Design review of the part built by this model. Coordinates are the model's own, in mm. Face numbers are marked on the shaded views. A direction names the side the tool comes from. Round coordinates to 2 decimals unless told otherwise and drop trailing zeros. Loops run counter-clockwise (first coordinate to the right, second up) from the corner with the lowest first, then second, coordinate; pieces in that order, holes last. Notation, with made-up numbers: (37, 69) - (90, 69) arc R31 ccw to (90, 97) - close; hole circle Ø4 at (-38, 5.5). An arc over 180 degrees is marked (long way). Answer as CSV lines item,"result". Start each with the question number.
(1) Wall thickness on L1, parallel to Z at x = 24.75, y = 7.25; L2, parallel to X at y = 1.5, z = -2; L3, parallel to X at y = 1.5, z = -66.5: over which ranges is each line inside the solid? List them lowest first.
(2) For P1, Ø2, axis at x = 9.5, y = 3, coming from the -Z side; P2, Ø3, axis at y = 4, z = -44.5, coming from the +X side; P3, Ø2, axis at y = 5, z = -30.5, coming from the -X side, all flat-tipped, find the tip position at first contact; note any pin that passes through.
(3) Consider section B-B (z = 2). Give the boundary of the cut face in (x, y).
(4) Consider section C-C (x = 24). Give the boundary of the cut face in (y, z).
(5) For the marked faces 1 and 2, list the 3-axis set-ups (+Z, -Z, +X, -X, +Y, -Y) from which the entire face can be reached by the end or side of a thin tool; tool diameter is ignored.
(6) Consider section A-A (y = 4.5). Give the boundary of the cut face in (x, z), and give its area (3 significant figures).
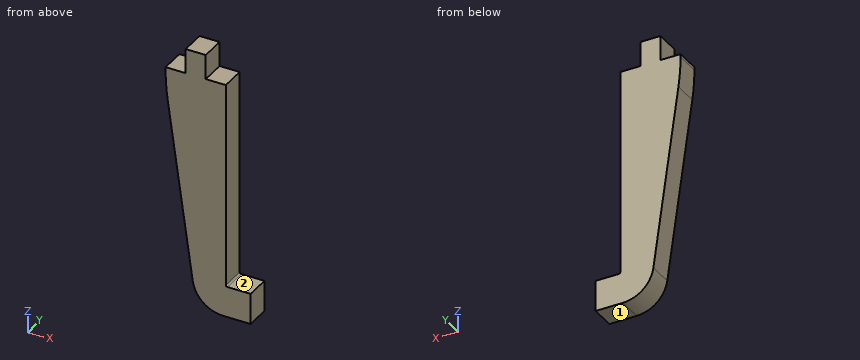
from build123d import *

# Parameters (mm, degrees)
BOSS_EXTRUDE1_DEPTH = 8
CHAMFER1_SIZE       = 10
CHAMFER1_SIZE2      = 71.153697224
FILLET1_R           = 10
FILLET2_R           = 70
FILLET3_R           = 0.5


with BuildPart() as part:
    # Sketch1 → Boss-Extrude1 (new body)
    with BuildSketch(Plane(origin=(0, 0, 0), x_dir=(1, 0, 0), z_dir=(0, 1, 0))):
        Polygon((0, 77), (0, 0), (6.5, 0), (6.5, -8), (13, -8), (13, 0), (19.5, 0), (19.5, 67), (27.5, 67), (27.5, 77), align=None)
    extrude(amount=BOSS_EXTRUDE1_DEPTH)

    # Chamfer1
    chamfer1_edges = [part.edges().sort_by_distance(p)[0] for p in [
        (0, 4, -77),
    ]]
    chamfer1_side = [part.faces().sort_by_distance(p)[0] for p in [
        (13.75, 4, -77),
    ]]
    chamfer(chamfer1_edges, length=CHAMFER1_SIZE, length2=CHAMFER1_SIZE2, reference=chamfer1_side[0])

    # Fillet1
    fillet1_edges = [part.edges().sort_by_distance(p)[0] for p in [
        (10, 4, -77),
    ]]
    fillet(fillet1_edges, radius=FILLET1_R)

    # Fillet2
    fillet2_edges = [part.edges().sort_by_distance(p)[0] for p in [
        (0, 4, -5.846302776),
    ]]
    fillet(fillet2_edges, radius=FILLET2_R)

    # Fillet3
    fillet3_edges = [part.edges().sort_by_distance(p)[0] for p in [
        (19.5, 4, -67),
    ]]
    fillet(fillet3_edges, radius=FILLET3_R)


solid = part.part
Determined:
1,L1,"z = -77 to -67"
1,L2,"x = 0.01 to 19.5"
1,L3,"x = 8.52 to 19.5"
2,P1,"stops at z = -72.73"
2,P2,"stops at x = 19.5"
2,P3,"stops at x = 3.32"
3,outline,"(6.5, 0) - (13, 0) - (13, 8) - (6.5, 8) - close"
4,outline,"(0, -77) - (8, -77) - (8, -67) - (0, -67) - close"
5,face 1,"-Z, +X, -X, +Y, -Y"
5,face 2,"+Z, +X, +Y, -Y"
6,outline,"(0, -0.95) arc R70 ccw to (0.68, -10.69) - (8.79, -68.39) arc R10 ccw to (18.69, -77) - (27.5, -77) - (27.5, -67) - (20, -67) arc R0.5 cw to (19.5, -66.5) - (19.5, 0) - (13, 0) - (13, 8) - (6.5, 8) - (6.5, 0) - (0, 0) - close"
6,area,"1,260 mm^2"
